Geometry check sheet. Reference: the model listing, model coordinates, mm. Face numbers are marked on the shaded views. A direction names the side the tool comes from. Give positions to 0.01 mm unless a question says otherwise; leave off trailing zeros. Loops run counter-clockwise (first coordinate to the right, second up) from the corner with the lowest first, then second, coordinate; pieces in that order, holes last.
1. Cross-section at D-D, the plane x = 70. Record the cut outline in (y, z).
2. Material ranges on L1, parallel to Z at x = 17.5, y = -23.25; L2, parallel to Z at x = 20, y = -22.5, recorded low to high.
3. Cross-section at A-A, the plane x = 105. Record the cut outline in (y, z), plus the area to 3 significant figures.
4. Go/stop test with a flat-tipped pin: pin 1 Ø10 at (x, z) = (100.98, 27.38) entering from -Y. Record where the tip stops, or that it passes through.
5. Cross-section at B-B, the plane y = -17.5. Record the cut outline in (x, z), plus the area to 3 significant figures.
6. Cross-section at C-C, the plane y = -3. Record the cut outline in (x, z).
7. Release check for a two-part mould opening along Z. For the marked faces 1, 2 and 3 record: +Z half, -Z half, draft (parallel to the pull), parting line (faces both ways), or undercut.
8. Tool access check on the marked faces 4 and 5. Record the directions out of +Z, -Z, +X, -X, +Y, -Y that give a thin tool (end or side, any length) a straight path to the whole face; none if there is none.
from build123d import *

# Parameters (mm, degrees)
F0_W           = 127
F0_H           = 50.8
F1_DEPTH       = 25.4
F3_D           = 12.7
F3_DEPTH       = 12.7
F3_CBORE_D     = 12.7
F3_CBORE_DEPTH = 6.35
F3_TIP         = 3.8154649308
F4_D           = 12.7
F5_D           = 12.7
F6_D           = 12.7


with BuildPart() as f1:
    # F0 (on Front) → F1 (new body)
    with BuildSketch(Plane.XZ):
        with Locations((63.5, 25.4)):
            Rectangle(F0_W, F0_H)
    extrude(amount=F1_DEPTH)

    # F3
    with Locations(Plane.XZ.offset(25.4)):
        with Locations((17.9662257433, 27.3820236325)):
            CounterBoreHole(F3_D / 2, F3_CBORE_D / 2, F3_CBORE_DEPTH, depth=F3_DEPTH)
            with Locations((0, 0, -(F3_DEPTH + F3_TIP / 2))):  # 118° drill point
                Cone(0, F3_D / 2, F3_TIP, mode=Mode.SUBTRACT)

    # F4 (through all)
    with Locations(Plane.XZ.offset(25.4)):
        with Locations((39.9235635996, 27.3820236325)):
            Hole(F4_D / 2)

    # F5 (through all)
    with Locations(Plane.XZ.offset(25.4)):
        with Locations((66.1182850599, 27.3820236325)):
            Hole(F5_D / 2)

    # F6 (through all)
    with Locations(Plane.XZ.offset(25.4)):
        with Locations((100.9803712368, 27.3820236325)):
            Hole(F6_D / 2)


solid = f1.part
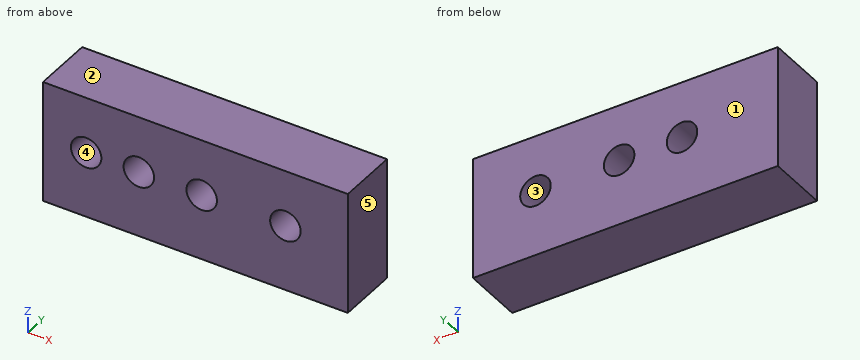
Result:
1. outline: (-25.4, 0) - (0, 0) - (0, 22.36) - (-25.4, 22.36) - close; (-25.4, 32.41) - (0, 32.41) - (0, 50.8) - (-25.4, 50.8) - close
2. L1: z = 0 to 21.05, 33.71 to 50.8
2. L2: z = 0 to 21.37, 33.4 to 50.8
3. outline: (-25.4, 0) - (0, 0) - (0, 22.47) - (-25.4, 22.47) - close; (-25.4, 32.3) - (0, 32.3) - (0, 50.8) - (-25.4, 50.8) - close
3. area: 1,040 mm2
4. pin 1: passes through
5. outline: (0, 0) - (127, 0) - (127, 50.8) - (0, 50.8) - close; hole circle Ø12.7 at (17.97, 27.38); hole circle Ø12.7 at (39.92, 27.38); hole circle Ø12.7 at (66.12, 27.38); hole circle Ø12.7 at (100.98, 27.38)
5. area: 5,940 mm2
6. outline: (0, 0) - (127, 0) - (127, 50.8) - (0, 50.8) - close; hole circle Ø12.7 at (39.92, 27.38); hole circle Ø12.7 at (66.12, 27.38); hole circle Ø12.7 at (100.98, 27.38)
7. face 1: draft
7. face 2: +Z half
7. face 3: undercut
8. face 4: -Y
8. face 5: +Z, -Z, +X, +Y, -Y
